The listing builds one solid part. Answer for the finished solid, in the listing's coordinates (mm). Coordinates: 2 decimals unless noted, no trailing zeros. Write each loop counter-clockwise with the first axis right and the second up, starting at its lowest first coordinate (ties: lowest second). Pieces come first, ordered by that corner, then holes. Notation, with made-up numbers: M 37,60 L 43,60 A18 ccw 43,79 Z; hole C -30.5,14 d1. An arc over 180 degrees is marked long. Answer as CSV lines item,"result".
```python
from build123d import *

# Parameters (mm, degrees)
F0_R     = 42.0549170166
F1_DEPTH = 12.954
F2_R     = 5.08
F4_R     = 30.1481321403
F5_DEPTH = 43.18
F6_R     = 36.9749170166
F7_DEPTH = 77.47
F8_R     = 36.9749170166
F9_DEPTH = 29.464


# Not quite as in the source:
# - a feature of the source that left no trace in its solid (it failed there, or was rolled back) is left out


with BuildPart() as f1:
    # F0 (on Top) → F1 (new body)
    with BuildSketch(Plane.XY):
        Circle(F0_R)
    extrude(amount=F1_DEPTH)

    # F2
    f2_edges = [f1.edges().sort_by_distance(p)[0] for p in [
        (-42.054917, 0, 12.954),
        (-42.054917, 0, 0),
    ]]
    fillet(f2_edges, radius=F2_R)

    # F4 (on Front) → F5 (join)
    with BuildSketch(Plane.XZ):
        with Locations((0, 21.2246719748)):
            Circle(F4_R)
    extrude(amount=F5_DEPTH)

    # F6 (on Top) → F7 (cut)
    with BuildSketch(Plane.XY):
        Circle(F6_R)
    extrude(amount=F7_DEPTH, mode=Mode.SUBTRACT)

    # F8 (on Top) → F9 (cut)
    with BuildSketch(Plane.XY):
        Circle(F8_R)
    extrude(amount=-F9_DEPTH, mode=Mode.SUBTRACT)


solid = f1.part
```
Q1. The mould has two halves that part along Y. Classify faces 1 (the cylindrical face through (1.47, 42.03, 6.46)), 2 (the flat face through (0, -43.18, 22)), 3 (the cylindrical face through (-8, -36.1, 14.1)): pulls with the +Y half, pulls with the -Y half, needs draft (parallel to the pull), parting line crosses it, or undercut.
Output:
face 1,"parting line crosses it"
face 2,"pulls with the -Y half"
face 3,"undercut"
Q2. Flat-ended cylindrical pins translate along their axes: pin 1 Ø6 at (x, y) = (29, -18.5) entering from +Z; pin 2 Ø6 at (y, z) = (8, 2.5) entering from -X; pin 3 Ø2 at (x, z) = (13.5, 18.5) entering from +Y. Find the tip coordinate at first contact, or state that the pin passes through.
Output:
pin 1,"z = 12.95"
pin 2,"x = -41.62"
pin 3,"y = -34.01"
Q3. Find section A-A (x = 0). Give the vertices of the cut face in (y, z), and give its area (3 significant figures).
Output:
outline,"M -43.18,-8.92 L -36.97,-8.92 L -36.97,51.37 L -43.18,51.37 Z; M 36.97,0 A5.08 ccw 42.05,5.08 L 42.05,7.87 A5.08 ccw 36.97,12.95 Z"
area,"429 mm2"
Q4. Straight lines are drawn through the part: line 1 (X direction, y = 0, z = 6); line 2 (Y direction, x = 0, z = 26); line 3 (X direction, y = 7, z = 8.5). For each, find the intervals that lie inside material, in ascending order.
Output:
line 1,"-42.05 to -36.97, 36.97 to 42.05"
line 2,"-43.18 to -36.97"
line 3,"-41.43 to -36.31, 36.31 to 41.43"
Q5. Find section C-C (z = -3.5). Give the vertices of the cut face in (x, y).
Output:
outline,"M -17.25,-43.18 L 17.25,-43.18 L 17.25,-32.7 A36.97 cw -17.25,-32.7 Z"
Q6. Find section B-B (z = 10.5). Give the vertices of the cut face in (x, y), and give its area (3 significant figures).
Output:
outline,"M -28.18,-43.18 L 28.18,-43.18 L 28.18,-30.23 A41.32 ccw long -28.18,-30.23 Z; hole C 0,0 d73.95"
area,"1,370 mm2"
